from build123d import *

# Parameters (mm, degrees)
SKETCH2_OUTSIDE_W  = 15.842
SKETCH2_OUTSIDE_H  = 15.842
CUT_EXTRUDE1_DEPTH = 10
SHELL1_T           = -1.5
CUT_EXTRUDE2_DEPTH = 11


with BuildPart() as part:
    # Sketch1 → Revolve1 (revolve)
    with BuildSketch(Plane.XY, mode=Mode.PRIVATE) as revolve1_sk:
        Polygon((0, 0), (0, 5), (2, 5), (2, 3.1), (13, 3.1), (13, 0), align=None)
    revolve(revolve1_sk.sketch.rotate(Axis((0, 0, 0), (1, 0, 0)), 90), axis=Axis((0, 0, 0), (1, 0, 0)))

    # Sketch2 outside → Cut-Extrude1 (cut)
    with BuildSketch(Plane.ZY):
        Rectangle(SKETCH2_OUTSIDE_W, SKETCH2_OUTSIDE_H)
        Polygon((0, -5), (4.330127019, -2.5), (4.330127019, 2.5), (0, 5), (-4.330127019, 2.5), (-4.330127019, -2.5), align=None, mode=Mode.SUBTRACT)
    extrude(amount=-CUT_EXTRUDE1_DEPTH, mode=Mode.SUBTRACT)

    # Shell1
    shell1_openings = [part.faces().sort_by_distance(p)[0] for p in [
        (13, 0, 0),
    ]]
    offset(amount=SHELL1_T, openings=shell1_openings, kind=Kind.INTERSECTION)

    # Sketch3 → Cut-Extrude2 (cut)
    with BuildSketch(Plane(origin=(13, 0, 0), x_dir=(0, 0, -1), z_dir=(1, 0, 0))):
        with BuildLine():
            Line((1.523154621, 2.7), (-1.523154621, 2.7))
            ThreePointArc((-1.523154621, 2.7), (0, 3.1), (1.523154621, 2.7))
        make_face()
    extrude(amount=-CUT_EXTRUDE2_DEPTH, mode=Mode.SUBTRACT)


solid = part.part
The listing builds one solid part. Answer for the finished solid, in the listing's coordinates (mm). A direction names the side the tool comes from. Coordinates: 2 decimals unless noted, no trailing zeros. Order: outer loops, then holes, each group sorted by start corner. A loop starts at its lowest first (then second) coordinate and runs counter-clockwise, first axis right, second up.
Q1. Given P1, Ø5, axis at x = 10, z = 3.5, coming from the -Y side; P2, Ø0.9, axis at x = 6.5, z = 0, coming from the +Y side; P3, Ø1, axis at y = -0.5, z = 0, coming from the +X side; P4, Ø5, axis at y = 0, z = 0, coming from the -X side, each flat-ended and moving along its own axis, determine where each tip first touches the part or whether it passes through.
Q2. A cutting plane is placed at A-A, the plane y = 0. Write down the section's boundary in (x, z).
Q3. Consider line 1 (Y direction, x = 6.75, z = 0); line 2 (X direction, y = -0.75, z = 1.25); line 3 (X direction, y = -1.5, z = 3.25). Determine where each line is inside the solid, lowest interval first.
Q4. A cutting plane is placed at C-C, the plane x = 2.5. Write down the section's boundary in (y, z).
Q5. A cutting plane is placed at B-B, the plane z = -0.75. Write down the section's boundary in (x, y).
Q6. A cutting plane is placed at D-D, the plane y = 2. Write down the section's boundary in (x, z).
Q7. For a pull along Z with two mould halves and no side action, classify faces 4 (the face through (0.99, 3.73, 2.2)), 5 (the face through (1.5, 0, 0)), 6 (the face through (7.6, -3.1, 0.1)), 7 (the face through (1, 0, -4.33)) as pulls with the +Z half, pulls with the -Z half, needs draft (parallel to the pull), parting line crosses it, or undercut.
Q8. Which of the six approach directions +Z, -Z, +X, -X, +Y, -Y give full straight-line access (tool end or side, diameter ignored) to faces 1 (the face through (8, 2.7, 0)), 2 (the face through (2, 3, 0)), 3 (the face through (0.99, 3.77, -2.13))?
Answers follow:
1. P1: stops at y = -2.93
1. P2: stops at y = 2.7
1. P3: stops at x = 1.5
1. P4: stops at x = 0
2. outline: (0, -4.33) - (2, -4.33) - (2, -3.1) - (13, -3.1) - (13, -1.6) - (1.5, -1.6) - (1.5, 1.6) - (13, 1.6) - (13, 3.1) - (2, 3.1) - (2, 4.33) - (0, 4.33) - close
3. line 1: y = -3.1 to -1.6, 1.6 to 2.7
3. line 2: x = 0 to 1.5
3. line 3: x = 0 to 2
4. outline: (2.7, -1.52) - (2.7, 1.52) arc R3.1 ccw (long way) to start; hole circle Ø3.2 at (0, 0)
5. outline: (0, -4.57) - (2, -4.57) - (2, -3.01) - (13, -3.01) - (13, -1.41) - (1.5, -1.41) - (1.5, 1.41) - (13, 1.41) - (13, 2.7) - (2, 2.7) - (2, 4.57) - (0, 4.57) - close
6. outline: (0, -4.33) - (2, -4.33) - (2, -2.37) - (13, -2.37) - (13, 2.37) - (2, 2.37) - (2, 4.33) - (0, 4.33) - close
7. face 4: pulls with the +Z half
7. face 5: undercut
7. face 6: parting line crosses it
7. face 7: pulls with the -Z half
8. face 1: +Z, -Z, +X, +Y
8. face 2: +X
8. face 3: -Z, +X, -X, +Y
